The listing builds one solid part. Answer for the finished solid, in the listing's coordinates (mm). A direction names the side the tool comes from. Give positions to 0.01 mm unless a question says otherwise; leave off trailing zeros. Loops run counter-clockwise (first coordinate to the right, second up) from the corner with the lowest first, then second, coordinate; pieces in that order, holes last. Notation, with made-up numbers: (-16.5, 63) - (7.5, 63) arc R8 cw to (7.5, 73) - close; hole circle Ø10 at (34.25, 36). An arc over 180 degrees is marked (long way). Write item = value, one per line. Start each with the question number.
1) The part is cut by section B-B on y = 17.5. Write down the section's boundary in (x, z), plus the area to 3 significant figures.
2) The part is cut by section D-D on x = 2. State how many separate pieces and enclosed holes the cut face has, plus the area to 3 significant figures.
3) The part is cut by section C-C on y = -14.5. Write down the section's boundary in (x, z).
4) Consider probe 1 along X at (y, z) = (-10, 8); probe 2 along Z at (x, y) = (15, -12); probe 3 along Z at (x, y) = (-6, 7.5). Determine where each line is inside the solid, lowest interval first.
5) The mould has two halves that part along Y. Classify faces 1 (the flat face through (0, 26, 0.5)), 2 (the flat face through (10, -24.892, 6)), 3 (the flat face through (0, 29.892, 2)): +Y half, -Y half, draft (parallel to the pull), parting line (faces both ways), or undercut.
6) Flat-ended cylindrical pins translate along their axes: P1, Ø15, axis at x = -3.5, y = -12, coming from the +Z side; P2, Ø6, axis at x = -4.5, y = 1, coming from the +Z side; P3, Ø2.5, axis at x = 16.47, y = -27.392, coming from the -Z side. Find the tip coordinate at first contact, or state that the pin passes through.
7) Which of the six approach directions +Z, -Z, +X, -X, +Y, -Y give full straight-line access (tool end or side, diameter ignored) to faces 4 (the flat face through (-9.72, -27, 6)), 5 (the flat face through (-13.97, 19, 3)), 6 (the flat face through (-12, -24.892, 6)), 7 (the cylindrical face through (15.364, -26.378, 9.014)), 8 (the conical face through (1.08, -14.97, 9.77))?
8) The part is cut by section A-A on x = 16.47. Write down the section's boundary in (y, z), plus the area to 3 significant figures.
from build123d import *

# Parameters (mm, degrees)
SKETCH002_W     = 37.94
SKETCH002_H     = 59.784
SKETCH002_R     = 1
SKETCH002_W_2   = 27.94
SKETCH002_H_2   = 49.784
PAD_DEPTH       = 10
POCKET_DEPTH    = 37.94
POCKET001_DEPTH = 37.94
PAD001_DEPTH    = 27.94
SKETCH005_W     = 33.575
SKETCH005_H     = 1
PAD002_DEPTH    = 27.94
SKETCH006_R     = 1.5
POCKET002_DEPTH = 2
SKETCH007_R     = 1.5
POCKET003_DEPTH = 2
SKETCH008_W     = 15.24
SKETCH008_H     = 5
POCKET004_DEPTH = 6
CONE_ANGLE      = 180
CONE001_ANGLE   = 180
CONE002_ANGLE   = 180
FILLET_R        = 0.75


with BuildPart() as part:
    # Sketch002 → Pad (new body)
    with BuildSketch(Plane.XY):
        Rectangle(SKETCH002_W, SKETCH002_H)
        with Locations((-16.47, 27.392)):
            Circle(SKETCH002_R, mode=Mode.SUBTRACT)
        with Locations((16.47, 27.392)):
            Circle(SKETCH002_R, mode=Mode.SUBTRACT)
        with Locations((-16.47, -27.392)):
            Circle(SKETCH002_R, mode=Mode.SUBTRACT)
        with Locations((16.47, -27.392)):
            Circle(SKETCH002_R, mode=Mode.SUBTRACT)
        Rectangle(SKETCH002_W_2, SKETCH002_H_2, mode=Mode.SUBTRACT)
    extrude(amount=PAD_DEPTH)

    # Sketch (on Face2 of Pad) → Pocket (cut)
    with BuildSketch(Plane.YZ.offset(18.97)):
        Polygon((8.683, 10), (29.892, 10), (29.892, 4.5), (14.183, 4.5), align=None)
        Polygon((-29.892, 4), (12.692, 4), (16.692, 0), (-29.892, 0), align=None)
    extrude(amount=-POCKET_DEPTH, mode=Mode.SUBTRACT)

    # Sketch003 (on Face3 of Pocket) → Pocket001 (cut)
    with BuildSketch(Plane.YZ.offset(18.97)):
        Polygon((16.192, 0.5), (29.892, 0.5), (29.892, 0), (16.692, 0), align=None)
    extrude(amount=-POCKET001_DEPTH, mode=Mode.SUBTRACT)

    # Sketch004 (on Face7 of Pocket001) → Pad001 (join)
    with BuildSketch(Plane.YZ.offset(-13.97)):
        Polygon((11.692, 7), (12.692, 6), (12.692, 4), (11.692, 4), align=None)
        Polygon((8.683, 10), (11.683, 7), (11.683, 6), (8.683, 9), align=None)
    extrude(amount=PAD001_DEPTH)

    # Sketch005 (on Face22 of Pad001) → Pad002 (join)
    with BuildSketch(Plane.YZ.offset(-13.97)):
        with Locations((-8.1045, 9.5)):
            Rectangle(SKETCH005_W, SKETCH005_H)
    extrude(amount=PAD002_DEPTH)

    # Sketch006 (on Face15 of Pad002) → Pocket002 (cut)
    with BuildSketch(Plane.XY.offset(10)):
        with Locations((-16.47, -27.392)):
            Circle(SKETCH006_R)
        with Locations((16.47, -27.392)):
            Circle(SKETCH006_R)
    extrude(amount=-POCKET002_DEPTH, mode=Mode.SUBTRACT)

    # Sketch007 (on Face4 of Pocket002) → Pocket003 (cut)
    with BuildSketch(Plane.XY.offset(4.5)):
        with Locations((-16.47, 27.392)):
            Circle(SKETCH007_R)
        with Locations((16.47, 27.392)):
            Circle(SKETCH007_R)
    extrude(amount=-POCKET003_DEPTH, mode=Mode.SUBTRACT)

    # Sketch008 (on Face15 of Pocket003) → Pocket004 (cut)
    with BuildSketch(Plane.XY.offset(10)):
        with Locations((-2.1, -27.392)):
            Rectangle(SKETCH008_W, SKETCH008_H)
    extrude(amount=-POCKET004_DEPTH, mode=Mode.SUBTRACT)

    # Cone → Cone (revolve, cut)
    with BuildSketch(Plane(origin=(-2.7, -4.892, 7), x_dir=(1, 0, 0), z_dir=(0, 0, -1))):
        Polygon((0, 0), (11.62, 25), (0, 25), align=None)
    revolve(axis=Axis((-2.7, -4.892, 7), (0, -1, 0)), revolution_arc=CONE_ANGLE, mode=Mode.SUBTRACT)

    # Cone001 → Cone001 (revolve)
    with BuildSketch(Plane(origin=(-2.7, -4.892, 10), x_dir=(1, 0, 0), z_dir=(0, 0, -1))):
        Polygon((0, 0), (11.62, 25), (0, 25), align=None)
    revolve(axis=Axis((-2.7, -4.892, 10), (0, -1, 0)), revolution_arc=CONE001_ANGLE)

    # Cone002 → Cone002 (revolve, cut)
    with BuildSketch(Plane(origin=(-2.7, -4.892, 10), x_dir=(1, 0, 0), z_dir=(0, 0, -1))):
        Polygon((0, 0), (10.62, 25), (0, 25), align=None)
    revolve(axis=Axis((-2.7, -4.892, 10), (0, -1, 0)), revolution_arc=CONE002_ANGLE, mode=Mode.SUBTRACT)

    # Fillet
    fillet_edges = [part.edges().sort_by_distance(p)[0] for p in [
        (-18.97, -29.892, 7),
        (18.97, -29.892, 7),
        (18.97, -10.6045, 10),
        (18.97, 11.433, 7.25),
        (18.97, 22.0375, 4.5),
        (0, 29.892, 4.5),
        (-18.97, 29.892, 2.5),
        (-18.97, 22.0375, 4.5),
        (18.97, 29.892, 2.5),
        (-18.97, 11.433, 7.25),
        (-18.97, -10.6045, 10),
        (-16.47, 8.683, 10),
        (0, 8.683, 10),
        (16.47, 8.683, 10),
    ]]
    fillet(fillet_edges, radius=FILLET_R)


solid = part.part
Answer below:
q1.outline = (-18.97, 0.5) - (-13.97, 0.5) - (-13.97, 4.5) - (-18.22, 4.5) arc R0.75 ccw to (-18.97, 3.75) - close; (13.97, 0.5) - (18.97, 0.5) - (18.97, 3.75) arc R0.75 ccw to (18.22, 4.5) - (13.97, 4.5) - close
q1.area = 39.8 mm2
q2.separate_pieces = 3
q2.enclosed_holes = 0
q2.area = 65.1 mm2
q3.outline = (-18.97, 4) - (-13.97, 4) - (-13.97, 9) - (-6.69, 9) arc R4.47 cw to (-6.01, 10) - (-6.78, 10) arc R4.08 cw to (1.38, 10) - (0.61, 10) arc R4.47 cw to (1.29, 9) - (13.97, 9) - (13.97, 4) - (18.97, 4) - (18.97, 9.25) arc R0.75 ccw to (18.22, 10) - (1.77, 10) arc R4.47 ccw to (-7.17, 10) - (-18.22, 10) arc R0.75 ccw to (-18.97, 9.25) - close
q4.probe_1 = -18.97 to -13.97, 13.97 to 18.97
q4.probe_2 = 4 to 10
q4.probe_3 = 9 to 10
q5.face_1 = draft
q5.face_2 = undercut
q5.face_3 = +Y half
q6.P1 = 16.78
q6.P2 = 10
q6.P3 = 4
q7.face_4 = -Z, -Y
q7.face_5 = +Z, -Z
q7.face_6 = -Z
q7.face_7 = +Z
q7.face_8 = -Y
q8.outline = (-29.89, 4) - (-28.39, 4) - (-28.39, 8) - (-28.89, 8) - (-28.89, 10) - (-29.89, 10) - close; (-26.39, 4) - (12.69, 4) - (16.19, 0.5) - (26.39, 0.5) - (26.39, 2.5) - (25.89, 2.5) - (25.89, 4.5) - (14.18, 4.5) - (8.9, 9.78) arc R0.75 ccw to (8.37, 10) - (-25.89, 10) - (-25.89, 8) - (-26.39, 8) - close; (28.39, 0.5) - (29.89, 0.5) - (29.89, 3.75) arc R0.75 ccw to (29.14, 4.5) - (28.89, 4.5) - (28.89, 2.5) - (28.39, 2.5) - close
q8.area = 287 mm2
